from build123d import *

# Parameters (mm, degrees)
BOSS_EXTRUDE1_DEPTH = 12.7
SKETCH3_R           = 2.032
CUT_EXTRUDE1_DEPTH  = 12.7


with BuildPart() as part:
    # Sketch1 → Boss-Extrude1 (new body)
    with BuildSketch(Plane.XY):
        with BuildLine():
            Line((-9.163521891, -0.002572295), (-9.163521891, -10.002577695))
            Line((-9.163521891, -10.002577695), (-21.863521891, -10.002577695))
            Line((-21.863521891, -10.002577695), (-21.863521891, -7.462577695))
            Line((-21.863521891, -7.462577695), (-11.703521891, -7.462577695))
            Line((-11.703521891, -7.462577695), (-11.703521891, -0.002572295))
            ThreePointArc((-11.703521891, -0.002572295), (0.836483509, 12.537433105), (13.376488909, -0.002572295))
            Line((13.376488909, -0.002572295), (13.376488909, -7.462577695))
            Line((13.376488909, -7.462577695), (23.536488909, -7.462577695))
            Line((23.536488909, -7.462577695), (23.536488909, -10.002577695))
            Line((23.536488909, -10.002577695), (10.836488909, -10.002577695))
            Line((10.836488909, -10.002577695), (10.836488909, -0.002572295))
            ThreePointArc((10.836488909, -0.002572295), (0.836483509, 9.997433105), (-9.163521891, -0.002572295))
        make_face()
    extrude(amount=BOSS_EXTRUDE1_DEPTH)

    # Sketch3 → Cut-Extrude1 (cut)
    with BuildSketch(Plane(origin=(0, -7.462577695, 0), x_dir=(1, 0, 0), z_dir=(0, 1, 0))):
        with Locations((-16.783521891, -6.35)):
            Circle(SKETCH3_R)
        with Locations((18.456488909, -6.35)):
            Circle(SKETCH3_R)
    extrude(amount=-CUT_EXTRUDE1_DEPTH, mode=Mode.SUBTRACT)


solid = part.part
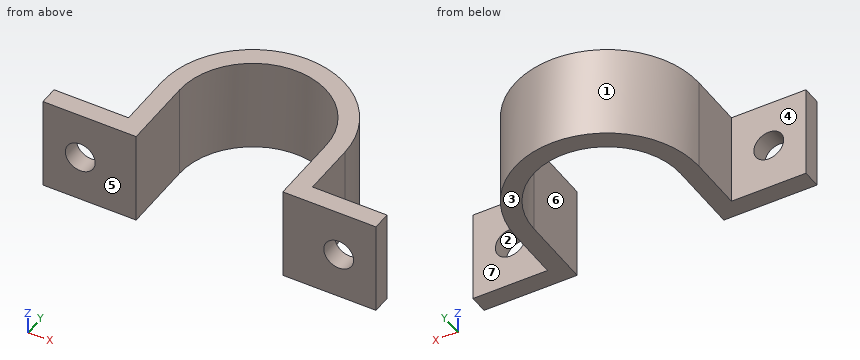
Can you work these out from the model? Positions are in its coordinate system, mm. Face numbers are marked on the shaded views. A direction names the side the tool comes from. Give positions to 0.01 mm unless a question says otherwise; leave off trailing zeros. Order: outer loops, then holes, each group sorted by start corner. A loop starts at its lowest first (then second) coordinate and runs counter-clockwise, first axis right, second up. Notation, with made-up numbers: (41, -6.75) - (52, -6.75) arc R22 cw to (52, 5.25) - close; hole circle Ø1 at (84, -3.75). An arc over 180 degrees is marked (long way). Write each question's results on one line, items separated by ' | '.
1) I'm going to push flat-ended pins straight in: pin 1 Ø4 at (x, z) = (-8.5, 4) entering from +Y; pin 2 Ø5 at (x, z) = (18.5, 4) entering from +Y; pin 3 Ø6 at (y, z) = (-2, 3) entering from +X. Where does each tip first touch, or does it pass through?
Final values:
pin 1: stops at y = 10.17 | pin 2: stops at y = -7.46 | pin 3: stops at x = 13.38
2) On a 3-axis mill with a long thin cutter (end or side, diameter ignored), from which of +Z, -Z, +X, -X, +Y, -Y can I reach the whole of each face in a straight line? I mean the marked faces 4, 5, 6 and 7. Say none if no direction works.
Final values:
face 4: +Z, -Z, -X, +Y | face 5: +Z, -Z, +X, -X, -Y | face 6: +Z, -Z, -Y | face 7: +Z, -Z, +X, +Y
3) Suppose I cut it at A-A, the plane y = -1.5. Write out the boundary of the cut face in (x, z).
Final values:
outline: (-11.7, 0) - (-9.16, 0) - (-9.16, 12.7) - (-11.7, 12.7) - close; (10.84, 0) - (13.38, 0) - (13.38, 12.7) - (10.84, 12.7) - close
4) Suppose I cut it at B-B, the plane z = 6.35. Write out the boundary of the cut face in (x, y), then the cut area to 3 significant figures.
Final values:
outline: (-21.86, -10) - (-18.82, -10) - (-18.82, -7.46) - (-21.86, -7.46) - close; (-14.75, -10) - (-9.16, -10) - (-9.16, 0) arc R10 cw to (10.84, 0) - (10.84, -10) - (16.42, -10) - (16.42, -7.46) - (13.38, -7.46) - (13.38, 0) arc R12.54 ccw to (-11.7, 0) - (-11.7, -7.46) - (-14.75, -7.46) - close; (20.49, -10) - (23.54, -10) - (23.54, -7.46) - (20.49, -7.46) - close | area: 172 mm^2
5) Suppose I cut it at C-C, the plane z = 2.5. Write out the boundary of the cut face in (x, y), then the cut area to 3 significant figures.
Final values:
outline: (-21.86, -10) - (-9.16, -10) - (-9.16, 0) arc R10 cw to (10.84, 0) - (10.84, -10) - (23.54, -10) - (23.54, -7.46) - (13.38, -7.46) - (13.38, 0) arc R12.54 ccw to (-11.7, 0) - (-11.7, -7.46) - (-21.86, -7.46) - close | area: 192 mm^2
6) Suppose I cut it at D-D, the plane y = 2.5. Write out the boundary of the cut face in (x, z).
Final values:
outline: (-11.45, 0) - (-8.85, 0) - (-8.85, 12.7) - (-11.45, 12.7) - close; (10.52, 0) - (13.12, 0) - (13.12, 12.7) - (10.52, 12.7) - close
7) Please list where these lines run through material, in increasing order: line 1 along X through (y, z) = (-8.9, 6.35); line 2 along X through (y, z) = (-2.25, 3.25); line 3 along Y through (x, z) = (-13, 4.25). Write a range as [from, to].
Final values:
line 1: x = [-21.86, -18.82], [-14.75, -9.16], [10.84, 16.42], [20.49, 23.54] | line 2: x = [-11.7, -9.16], [10.84, 13.38] | line 3: y = [-10, -7.46]
8) If we mould it in two halves opening along X, with no side actions, what happens to the marked faces 1, 2 and 3? For each: pulls with the +X half, pulls with the -X half, needs draft (parallel to the pull), parting line crosses it, or undercut.
Final values:
face 1: parting line crosses it | face 2: undercut | face 3: needs draft
